```python
from build123d import *

# Parameters (mm, degrees)
F0_R          = 13
F1_DEPTH      = 5
F2_R          = 10.5
F3_DEPTH      = 25
F3_DEPTH_BACK = 110
F6_START      = -19
F5_R          = 11.5
F5_R_2        = 10.5
F6_DEPTH      = 4
F7_R          = 11
F7_R_2        = 10.5
F8_DEPTH      = 15
F10_DEPTH     = 9
F11_R         = 1
F12_W         = 8.5742305964
F12_H         = 3.8462157547
F13_DEPTH     = 30
F14_T4_ANGLE  = 233.385278584
F16_START     = -15
F15_R         = 12.5
F15_R_2       = 10.5
F16_DEPTH     = 4
F18_START     = -11
F17_R         = 11
F17_R_2       = 10.5
F18_DEPTH     = 3
F19_R         = 2.75
F20_DEPTH     = 148


# Not quite as in the source:
# - a fillet or chamfer that OpenCascade refuses, or shapes differently, is made with other operations: its cross-section is extruded or revolved along the edge and cut away or added


with BuildPart() as f1:
    # F0 (on Front) → F1 (new body)
    with BuildSketch(Plane.XZ):
        Circle(F0_R)
    extrude(amount=F1_DEPTH)

    # F2 (on face) → F3 (join, two sides)
    with BuildSketch(Plane.XZ.offset(5)) as f3_sk:
        Circle(F2_R)
    extrude(amount=F3_DEPTH)
    extrude(f3_sk.sketch, amount=-F3_DEPTH_BACK)

    # F5 (on face) → F6 (join)
    with BuildSketch(Plane(origin=(0, 105, 0), x_dir=(-1, 0, 0), z_dir=(0, 1, 0)).offset(F6_START)):
        Circle(F5_R)
        Circle(F5_R_2, mode=Mode.SUBTRACT)
    extrude(amount=-F6_DEPTH)

    # F7 (on face) → F8 (join)
    with BuildSketch(Plane.XZ.offset(30)):
        Circle(F7_R)
        Circle(F7_R_2, mode=Mode.SUBTRACT)
    extrude(amount=-F8_DEPTH)

    # F9 (on face) → F10 (cut)
    with BuildSketch(Plane.XZ.offset(30)):
        with BuildLine():
            Line((-1.2941175373, 2.1176473238), (-1.2941175373, 10.9243700281))
            ThreePointArc((-1.2941175373, 10.9243700281), (-7.5067341919, 8.0813904617), (-10.8403367922, 2.1176473238))
            Line((-10.8403367922, 2.1176473238), (-1.2941175373, 2.1176473238))
        make_face()
    extrude(amount=-F10_DEPTH, mode=Mode.SUBTRACT)

    # F11
    f11_edges = [f1.edges().sort_by_distance(p)[0] for p in [
        (-6.044178, -21, 2.117647),
        (-1.294118, -21, 6.520629),
    ]]
    fillet(f11_edges, radius=F11_R)

    # F12 (on face) → F13 (cut)
    with BuildSketch(Plane.XY.offset(2.1176473238)):
        with Locations((-9.7801117226, -28.0768921226)):
            Rectangle(F12_W, F12_H)
    extrude(amount=-F13_DEPTH, mode=Mode.SUBTRACT)

    # F14: chamfer of 6 x 2 on 1 edges, made by hand


with BuildPart() as f14_tool2:
    # F14_s3 → F14_t4 (revolve)
    with BuildSketch(Plane(origin=(0, 0, 0), x_dir=(0, 1, 0), z_dir=(0.9992485549, 0, -0.0387598451))):
        Polygon((-24.1537842453, 11), (-26.1537842453, 5), (-26.1537842453, 11), align=None)
    revolve(axis=Axis((0, -26.1537842453, 0), (0, -1, 0)), revolution_arc=F14_T4_ANGLE)

    split(bisect_by=Plane.YZ.offset(-5.4929964244), keep=Keep.BOTTOM)


with BuildPart() as f1_1:
    add(f1.part)

    # F14_t1: cut F14_tool2
    add(f14_tool2.part, mode=Mode.SUBTRACT)

    # F15 (on face) → F16 (join)
    with BuildSketch(Plane(origin=(0, 105, 0), x_dir=(-1, 0, 0), z_dir=(0, 1, 0)).offset(F16_START)):
        Circle(F15_R)
        Circle(F15_R_2, mode=Mode.SUBTRACT)
    extrude(amount=-F16_DEPTH)

    # F17 (on face) → F18 (join)
    with BuildSketch(Plane(origin=(0, 105, 0), x_dir=(-1, 0, 0), z_dir=(0, 1, 0)).offset(F18_START)):
        Circle(F17_R)
        Circle(F17_R_2, mode=Mode.SUBTRACT)
    extrude(amount=-F18_DEPTH)

    # F19 (on face) → F20 (cut)
    with BuildSketch(Plane.XZ.offset(30)):
        with Locations((1.3252417254, -0.3058710963)):
            Circle(F19_R)
    extrude(amount=-F20_DEPTH, mode=Mode.SUBTRACT)


solid = f1_1.part
```
Geometry: final body of the model. Coordinates: model frame, mm. A direction names the side the tool comes from. Coordinates: 2 decimals unless noted, no trailing zeros. Order: outer loops, then holes, each group sorted by start corner. A loop starts at its lowest first (then second) coordinate and runs counter-clockwise, first axis right, second up. Notation, with made-up numbers: (46.5, -8) - (56.5, -8) arc R16 cw to (56.5, -3) - close; hole circle Ø8 at (45.5, 33). An arc over 180 degrees is marked (long way). Return JSON: item names as keys, results as strings. Group by question number.
1. Material intervals for line 1 along Y through (x, z) = (10.5, 4); line 2 along Z through (x, y) = (0.75, -4); line 3 along Z through (x, y) = (2, 56.5), sorted ascending. Write a range as [from, to].
2. Cut plane A-A (y = 50). Output: boundary loops of the cut face in (x, z), plus the area to 3 significant figures.
3. Pull-direction query (Y, two-part tool) for faces 5 (the face through (10, -9.9, 3.2)), 6 (the face through (4.5, -30, 0.2)), 7 (the face through (2.38, 92.52, -10.74)); classes: pulls with the +Y half, pulls with the -Y half, needs draft (parallel to the pull), parting line crosses it, or undercut.
4. Set-up query: faces 1 (the face through (-4, 94, -10)), 2 (the face through (-5, -25, 2.118)), 3 (the face through (-10.316, -2.465, -7.91)), 4 (the face through (-9, -5, 6)). Return all of +Z, -Z, +X, -X, +Y, -Y with unobstructed straight access to the full face (end or side cutting, diameter ignored); none if empty.
5. Pin query (flat end, axial travel): pin 1 (4 mm diameter, centred on x = -8, z = 4, fed in from -Y); pin 2 (4 mm diameter, centred on x = -6.5, z = 6, fed in from -Y); pin 3 (6 mm diameter, centred on y = 16, z = -2, fed in from +X); pin 4 (6 mm diameter, centred on y = -0.5, z = -3, fed in from -X). Return the tip coordinate at first contact, or that it passes through.
Resolved:
{
 "1": {"line 1": "y = [-5, 0], [82, 90]", "line 2": "z = [-12.98, -3], [2.38, 12.98]", "line 3": "z = [-10.31, -2.97], [2.36, 10.31]"},
 "2": {"outline": "circle Ø21 at (0, 0); hole circle Ø5.5 at (1.33, -0.31)", "area": "323 mm²"},
 "3": {"face 5": "undercut", "face 6": "pulls with the -Y half", "face 7": "needs draft"},
 "4": {"face 1": "+Y", "face 2": "+Z, -X, -Y", "face 3": "+Y, -Y", "face 4": "none"},
 "5": {"pin 1": "stops at y = -25.28", "pin 2": "stops at y = -21", "pin 3": "stops at x = 10.5", "pin 4": "stops at x = -13"}
}
